Geometry check sheet. Reference: the model listing, model coordinates, mm. Give positions to 0.01 mm unless a question says otherwise; leave off trailing zeros. Loops run counter-clockwise (first coordinate to the right, second up) from the corner with the lowest first, then second, coordinate; pieces in that order, holes last. Notation, with made-up numbers: (-26, -7) -> (-4, -7) arc R14 cw to (-4, 10) -> close; hole circle Ø3 at (33.25, 19.5). An arc over 180 degrees is marked (long way). Answer as a JSON object with one key per item and string values.
from build123d import *

# Parameters (mm, degrees)
SKETCH_1_R          = 1
EXTRUDE_1_DEPTH     = 4
CUT_EXTRUDE_1_DEPTH = 0.8
CHAMFER_1_SIZE      = 0.1


with BuildPart() as part:
    # 草图1 → 凸台-拉伸1 (new, symmetric)
    with BuildSketch(Plane.XY):
        Circle(SKETCH_1_R)
    extrude(amount=EXTRUDE_1_DEPTH, both=True)

    # 草图2 → 切除-拉伸1 (cut)
    with BuildSketch(Plane.XY.offset(4)):
        Polygon((0.259807621, 0.45), (-0.259807621, 0.45), (-0.519615242, 0), (-0.259807621, -0.45), (0.259807621, -0.45), (0.519615242, 0), align=None)
    extrude(amount=-CUT_EXTRUDE_1_DEPTH, mode=Mode.SUBTRACT)

    # 倒角1
    chamfer_1_edges = [part.edges().sort_by_distance(p)[0] for p in [
        (-1, 0, -4),
        (-1, 0, 4),
    ]]
    chamfer(chamfer_1_edges, length=CHAMFER_1_SIZE)


solid = part.part
1) Draft check along X on faces 1 (the face through (0, 0, 3.2)), 2 (the face through (0, 0, -4)), 3 (the face through (0, -1, 0)). Enter one of: pulls with the +X half, pulls with the -X half, needs draft (parallel to the pull), parting line crosses it, or undercut.
Geometry check:
{"face 1": "undercut", "face 2": "needs draft", "face 3": "parting line crosses it"}
2) Section check A-A on x = 0. Record the cut outline in (y, z), plus the area to 3 significant figures.
Geometry check:
{"outline": "(-1, -3.9) -> (-0.9, -4) -> (0.9, -4) -> (1, -3.9) -> (1, 3.9) -> (0.9, 4) -> (0.45, 4) -> (0.45, 3.2) -> (-0.45, 3.2) -> (-0.45, 4) -> (-0.9, 4) -> (-1, 3.9) -> close", "area": "15.3 mm2"}
3) Material ranges on line 1 along Z through (x, y) = (-0.2, -0.1); line 2 along X through (y, z) = (-0.65, -1.25); line 3 along Y through (x, z) = (0.2, 2.5), recorded low to high. Write a range as from..to.
Geometry check:
{"line 1": "z = -4..3.2", "line 2": "x = -0.76..0.76", "line 3": "y = -0.98..0.98"}
4) Section check B-B on z = -2.25. Record the cut outline in (x, y), plus the area to 3 significant figures.
Geometry check:
{"outline": "circle Ø2 at (0, 0)", "area": "3.14 mm2"}
